CAD build for the part. Positions are in the model's coordinates, mm. Face numbers are marked on the shaded views. Give positions to 0.01 mm unless a question says otherwise; leave off trailing zeros. Write each loop counter-clockwise with the first axis right and the second up, starting at its lowest first coordinate (ties: lowest second). Pieces come first, ordered by that corner, then holes. Notation, with made-up numbers: (83, 80) - (122, 80) arc R17 cw to (122, 87) - close; hole circle Ø5 at (-1, 79). An arc over 180 degrees is marked (long way). Answer as a JSON object with one key per item and string values.
from build123d import *

# Parameters (mm, degrees)
CROQUIS2_W              = 60
CROQUIS2_H              = 96.7
CROQUIS2_R              = 1.825
SALIENTE_EXTRUIR1_DEPTH = 5.5
REDONDEO2_R             = 5
CROQUIS4_R              = 39.5
CORTAR_EXTRUIR1_DEPTH   = 2.5
CROQUIS5_R              = 1.825
CORTAR_EXTRUIR2_DEPTH   = 114.841512639
CROQUIS6_R              = 3.325
CORTAR_EXTRUIR3_DEPTH   = 2.5
CROQUIS7_R              = 3.075
CORTAR_EXTRUIR4_DEPTH   = 3
CROQUIS10_R             = 40.2
CORTAR_EXTRUIR5_DEPTH   = 2.5


with BuildPart() as part:
    # Croquis2 → Saliente-Extruir1 (new body)
    with BuildSketch(Plane(origin=(0, 0, 0), x_dir=(1, 0, 0), z_dir=(0, 1, 0))):
        with Locations((30, 48.35)):
            Rectangle(CROQUIS2_W, CROQUIS2_H)
        with Locations(Location((9, 6.6, 0), (0, 0, 270))):
            Circle(CROQUIS2_R, mode=Mode.SUBTRACT)
        with Locations(Location((51, 6.6, 0), (0, 0, 270))):
            Circle(CROQUIS2_R, mode=Mode.SUBTRACT)
        with Locations(Location((9, 90.1, 0), (0, 0, 90))):
            Circle(CROQUIS2_R, mode=Mode.SUBTRACT)
        with Locations(Location((51, 90.1, 0), (0, 0, 90))):
            Circle(CROQUIS2_R, mode=Mode.SUBTRACT)
    extrude(amount=SALIENTE_EXTRUIR1_DEPTH)

    # Redondeo2
    redondeo2_edges = [part.edges().sort_by_distance(p)[0] for p in [
        (0, 2.75, -96.7),
        (60, 2.75, -96.7),
        (60, 2.75, 0),
        (0, 2.75, 0),
    ]]
    fillet(redondeo2_edges, radius=REDONDEO2_R)

    # Croquis4 → Cortar-Extruir1 (cut)
    with BuildSketch(Plane(origin=(0, 5.5, 0), x_dir=(1, 0, 0), z_dir=(0, 1, 0))):
        with Locations((22, 48.35)):
            Circle(CROQUIS4_R)
    extrude(amount=-CORTAR_EXTRUIR1_DEPTH, mode=Mode.SUBTRACT)

    # Croquis5 → Cortar-Extruir2 (cut, through all)
    with BuildSketch(Plane(origin=(0, 3, 0), x_dir=(1, 0, 0), z_dir=(0, 1, 0))):
        with Locations(Location((45.211409163, 69.352226887, 0), (0, 0, 270))):
            Circle(CROQUIS5_R)
        with Locations(Location((45.497544097, 27.633908047, 0), (0, 0, 270))):
            Circle(CROQUIS5_R)
    extrude(amount=-CORTAR_EXTRUIR2_DEPTH, mode=Mode.SUBTRACT)

    # Croquis6 → Cortar-Extruir3 (cut)
    with BuildSketch(Plane.XZ):
        with Locations(Location((45.497544097, -27.633908047, 0), (0, 0, 270))):
            Circle(CROQUIS6_R)
        with Locations(Location((45.211409163, -69.352226887, 0), (0, 0, 270))):
            Circle(CROQUIS6_R)
    extrude(amount=-CORTAR_EXTRUIR3_DEPTH, mode=Mode.SUBTRACT)

    # Croquis7 → Cortar-Extruir4 (cut)
    with BuildSketch(Plane(origin=(0, 5.5, 0), x_dir=(1, 0, 0), z_dir=(0, 1, 0))):
        with Locations(Location((51, 90.1, 0), (0, 0, 270))):
            Circle(CROQUIS7_R)
        with Locations(Location((9, 90.1, 0), (0, 0, 90))):
            Circle(CROQUIS7_R)
        with Locations(Location((51, 6.6, 0), (0, 0, 90))):
            Circle(CROQUIS7_R)
        with Locations(Location((9, 6.6, 0), (0, 0, 270))):
            Circle(CROQUIS7_R)
    extrude(amount=-CORTAR_EXTRUIR4_DEPTH, mode=Mode.SUBTRACT)

    # Croquis10 → Cortar-Extruir5 (cut)
    with BuildSketch(Plane(origin=(0, 5.5, 0), x_dir=(1, 0, 0), z_dir=(0, 1, 0))):
        with Locations((22, 48.35)):
            Circle(CROQUIS10_R)
    extrude(amount=-CORTAR_EXTRUIR5_DEPTH, mode=Mode.SUBTRACT)


solid = part.part
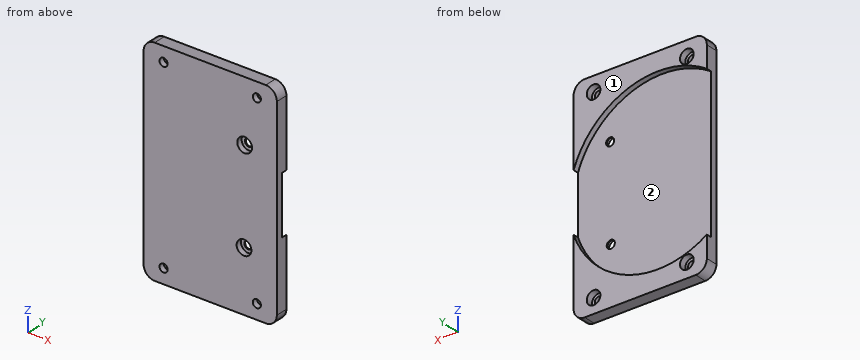
(1) Pull direction Z, two halves, no side cores. Call the marked faces 1 and 2: pulls with the +Z half, pulls with the -Z half, needs draft (parallel to the pull), parting line crosses it, or undercut.
Answer key:
{"face 1": "needs draft", "face 2": "undercut"}
(2) Probe L1, parallel to X at y = 1.1, z = -6.6 (3 decimals); L2, parallel to Z at x = 51, y = 0.65 (3 decimals); L3, parallel to X at y = 4.55, z = -90.1 (3 decimals). List the from-to ranges inside material, lowest first. Write a range as [from, to].
Answer key:
{"L1": "x = [0, 7.175], [10.825, 49.175], [52.825, 60]", "L2": "z = [-96.7, -91.925], [-88.275, -8.425], [-4.775, 0]", "L3": "x = [0, 5.925], [12.075, 47.925], [54.075, 60]"}
(3) Saw through at D-D, the plane z = -37. Give the cut face in (x, y), and give its area (3 significant figures).
Answer key:
{"outline": "(0, 0) - (60, 0) - (60, 3) - (0, 3) - close", "area": "180 mm²"}
(4) Flat gauge pins, fed straight in: P1, Ø6, axis at x = 51, z = -6.6, coming from the +Y side; P2, Ø7.5, axis at x = 45.5, z = -27.63, coming from the +Y side; P3, Ø6, axis at x = 45.5, z = -27.63, coming from the -Y side. Where does each tip first touch, or does it go through?
Answer key:
{"P1": "stops at y = 2.5", "P2": "stops at y = 3", "P3": "stops at y = 2.5"}
(5) Saw through at A-A, the plane z = -6.6. Give the cut face in (x, y) (3 decimals), and give its area (3 significant figures).
Answer key:
{"outline": "(0, 0) - (7.175, 0) - (7.175, 2.5) - (5.925, 2.5) - (5.925, 5.5) - (0, 5.5) - close; (10.825, 0) - (49.175, 0) - (49.175, 2.5) - (47.925, 2.5) - (47.925, 5.5) - (12.075, 5.5) - (12.075, 2.5) - (10.825, 2.5) - close; (52.825, 0) - (60, 0) - (60, 5.5) - (54.075, 5.5) - (54.075, 2.5) - (52.825, 2.5) - close", "area": "275 mm²"}
(6) Saw through at B-B, the plane x = 22. Give the cut face in (y, z), and give its area (3 significant figures).
Answer key:
{"outline": "(0, -96.7) - (5.5, -96.7) - (5.5, -88.55) - (3, -88.55) - (3, -8.15) - (5.5, -8.15) - (5.5, 0) - (0, 0) - close", "area": "331 mm²"}
(7) Saw through at C-C, the plane x = 9. Give the cut face in (y, z) (3 decimals).
Answer key:
{"outline": "(0, -96.7) - (5.5, -96.7) - (5.5, -93.175) - (2.5, -93.175) - (2.5, -91.925) - (0, -91.925) - close; (0, -88.275) - (2.5, -88.275) - (2.5, -87.025) - (5.5, -87.025) - (5.5, -86.39) - (3, -86.39) - (3, -10.31) - (5.5, -10.31) - (5.5, -9.675) - (2.5, -9.675) - (2.5, -8.425) - (0, -8.425) - close; (0, -4.775) - (2.5, -4.775) - (2.5, -3.525) - (5.5, -3.525) - (5.5, 0) - (0, 0) - close"}
